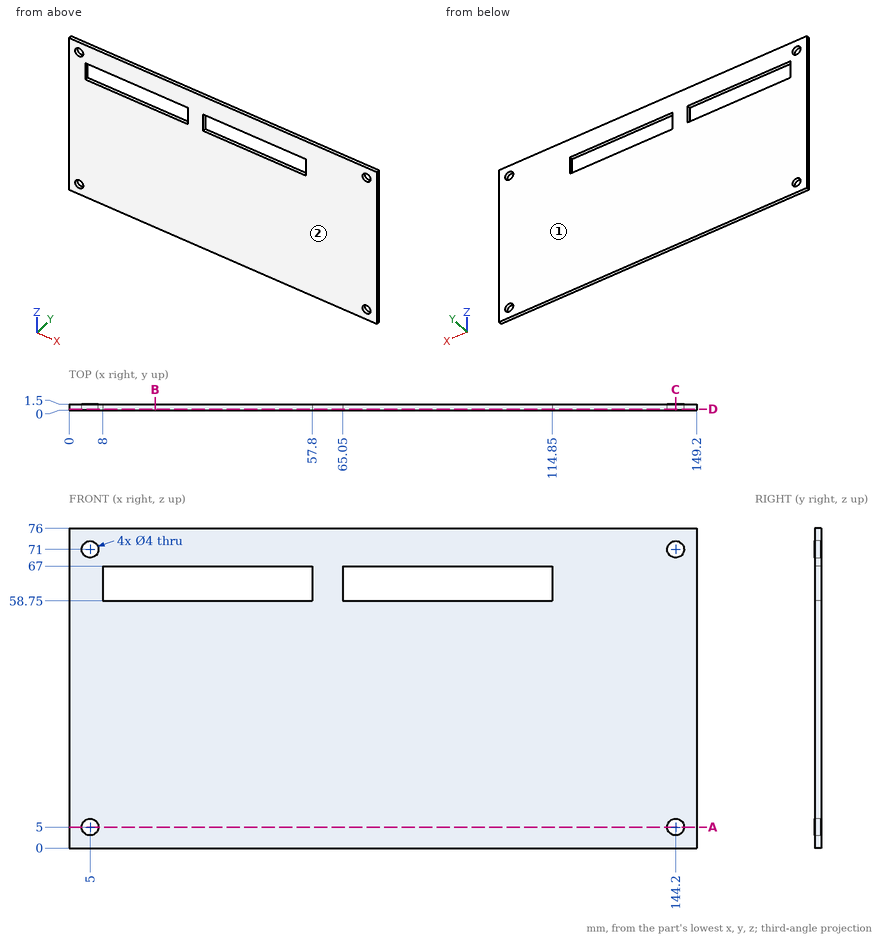
Design review of the part shown in the three views and the two pictorial views. Dimensions are in mm from the part's minimum x, y and z. Coordinates: 2 decimals unless noted, no trailing zeros. Order: outer loops, then holes, each group sorted by start corner. A loop starts at its lowest first (then second) coordinate and runs counter-clockwise, first axis right, second up. Notation, with made-up numbers: (77.5, 19) - (84.5, 19) arc R18 ccw to (84.5, 31) - close; hole circle Ø1 at (-29.5, 45). An arc over 180 degrees is marked (long way). Answer as CSV lines item,"result". Start each with the question number.
1) Insertion check: P1, Ø3.5, axis at x = 144.2, z = 5, coming from the +Y side. The pin has a flat end and moves straight along its axis. Give the tip position at first contact, or say it passes through.
2) Add section C-C (x = 144.2). State the section outline as (y, z) points.
3) Add section A-A (z = 5). State the section outline as (x, y) points.
4) Add section D-D (y = 0.3). State the section outline as (x, z) points.
5) Draft analysis for pull direction Y (two halves, no side actions). For the marked faces 1 and 2, state which applies: +Y half, -Y half, draft (parallel to the pull), parting line (faces both ways), or undercut.
6) Add section B-B (x = 20.5). State the section outline as (y, z) points, then the cut area to 3 significant figures.
7) To check wall thickness, follow line 1 along X through (y, z) = (0.4, 63.5); line 2 along X through (y, z) = (1, 5); line 3 along Z through (x, y) = (144.2, 0.45). State the ranges of each line that lie inside material, in increasing order. Write a range as [from, to].
Result:
1,P1,"through"
2,outline,"(0, 0) - (1.5, 0) - (1.5, 3) - (0, 3) - close; (0, 7) - (1.5, 7) - (1.5, 69) - (0, 69) - close; (0, 73) - (1.5, 73) - (1.5, 76) - (0, 76) - close"
3,outline,"(0, 0) - (3, 0) - (3, 1.5) - (0, 1.5) - close; (7, 0) - (142.2, 0) - (142.2, 1.5) - (7, 1.5) - close; (146.2, 0) - (149.2, 0) - (149.2, 1.5) - (146.2, 1.5) - close"
4,outline,"(0, 0) - (149.2, 0) - (149.2, 76) - (0, 76) - close; hole circle Ø4 at (5, 5); hole circle Ø4 at (5, 71); hole (8, 58.75) - (57.8, 58.75) - (57.8, 67) - (8, 67) - close; hole (65.05, 58.75) - (114.85, 58.75) - (114.85, 67) - (65.05, 67) - close; hole circle Ø4 at (144.2, 5); hole circle Ø4 at (144.2, 71)"
5,face 1,"+Y half"
5,face 2,"-Y half"
6,outline,"(0, 0) - (1.5, 0) - (1.5, 58.75) - (0, 58.75) - close; (0, 67) - (1.5, 67) - (1.5, 76) - (0, 76) - close"
6,area,"102 mm^2"
7,line 1,"[0, 8], [57.8, 65.05], [114.85, 149.2]"
7,line 2,"[0, 3], [7, 142.2], [146.2, 149.2]"
7,line 3,"[0, 3], [7, 69], [73, 76]"
